Check sheet for the modelled part. Datum: model origin and axes. Units: mm. Coordinates: 2 decimals unless noted, no trailing zeros. Loops run counter-clockwise (first coordinate to the right, second up) from the corner with the lowest first, then second, coordinate; pieces in that order, holes last. Notation, with made-up numbers: M -32,81 L 8,81 A18 ccw 8,103 Z; hole C 18.5,41 d9. An arc over 180 degrees is marked long. Use CSV: the item, a comma, the result in double quotes. Start each with the question number.
(1) Go/stop test with a flat-tipped pin: pin 1 Ø6 at (x, y) = (18, 1) entering from -Z. Record where the tip stops, or that it passes through.
(2) Section check B-B on y = 2.25. Record the cut outline in (x, z).
(3) Scan lines: line 1 (Y direction, x = 14, z = -23); line 2 (Z direction, x = -71, y = 2.25). Record each from-to range of solid material in increasing order.
(4) Section check C-C on z = -18.5. Record the cut outline in (x, y), and give its area (3 significant figures).
(5) Section check A-A on x = -16. Record the cut outline in (y, z).
from build123d import *

# Parameters (mm, degrees)
F0_W     = 170
F0_H     = 122.3707973333
F1_DEPTH = 5
F2_R     = 1.5
F3_DEPTH = 5


# Not quite as in the source:
# - a pattern or mirror of a feature is missing from the dataset's text; its kind, count and spacing are read off the source's solid


with BuildPart() as f1:
    # F0 (on Front) → F1 (new body)
    with BuildSketch(Plane.XZ):
        Rectangle(F0_W, F0_H)
    extrude(amount=F1_DEPTH)

    # F2 (on Front) → F3 (join)
    with BuildSketch(Plane.XZ):
        with Locations((70, 56.1853986666)):
            Circle(F2_R)
    f3 = extrude(amount=-F3_DEPTH)

    # F3_copies: F3 across plane
    add(f3.mirror(Plane(origin=(0, 0, 0), x_dir=(0, 0, -1), z_dir=(-1, 0, 0))))

    # F3_copies1: F3 across plane
    add(f3.mirror(Plane(origin=(0, 0, 0), x_dir=(-1, 0, 0), z_dir=(0, 0, -1))))

    # F3_copies2: F3 across plane
    add(f3.mirror(Plane(origin=(0, 0, 0), x_dir=(0.6259536866, 0, -0.7798602325), z_dir=(-0.7798602325, 0, -0.6259536866))))


solid = f1.part
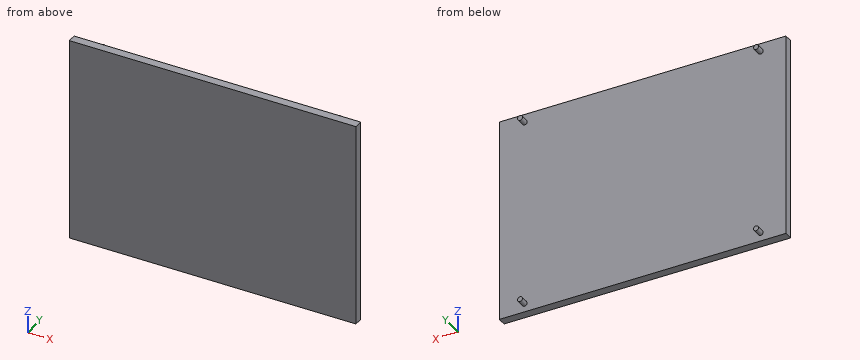
Outcome:
1,pin 1,"stops at z = -61.19"
2,outline,"C -70,-56.19 d3; C -70,56.19 d3; C 70,-56.19 d3; C 70,56.19 d3"
3,line 1,"y = -5 to 0"
3,line 2,"z = -57.3 to -55.07, 55.07 to 57.3"
4,outline,"M -85,-5 L 85,-5 L 85,0 L -85,0 Z"
4,area,"850 mm²"
5,outline,"M -5,-61.19 L 0,-61.19 L 0,61.19 L -5,61.19 Z"
